```python
from build123d import *

# Parameters (mm, degrees)
F0_W     = 117.000002
F0_H     = 72.900005
F1_DEPTH = 25
F4_D     = 5.5
F5_R     = 9.5
F6_DEPTH = 40


with BuildPart() as f1:
    # F0 (on Front) → F1 (new body)
    with BuildSketch(Plane.XZ):
        with Locations((-1.050001, 2.849999)):
            Rectangle(F0_W, F0_H)
    extrude(amount=F1_DEPTH)

    # F4 (through all)
    with Locations(Plane(origin=(48.375001, 0, 48.375001), x_dir=(0.707107, 0, -0.707107), z_dir=(0.707107, 0, 0.707107))):
        with Locations((13.142212, -14.138062)):
            Hole(F4_D / 2)

    # F5 (on face) → F6 (cut)
    with BuildSketch(Plane.XZ.offset(25)):
        with Locations((-39.750002, -15.600001)):
            Circle(F5_R)
    extrude(amount=-F6_DEPTH, mode=Mode.SUBTRACT)


solid = f1.part
```
Geometry: final body of the model. Coordinates: model frame, mm. Round coordinates to 2 decimals unless told otherwise and drop trailing zeros. Loops run counter-clockwise (first coordinate to the right, second up) from the corner with the lowest first, then second, coordinate; pieces in that order, holes last.
Item 1: Mould query, pull axis Y, two halves, no side actions, for faces 1 (the flat face through (-2, 0, 3)), 2 (the cylindrical face through (17.98, -13.31, 3.1)), 3 (the cylindrical face through (-49.24, -12.68, -15.18)). Classes: released by +Y, released by -Y, zero draft, split by the parting line, or undercut.
Checked values:
face 1: released by +Y
face 2: undercut
face 3: zero draft
Item 2: Section A-A, the plane y = -12.75. Output: boundary loops of the cut face in (x, z), plus the area to 3 significant figures.
Checked values:
outline: (-59.55, -33.6) - (-18.37, -33.6) - (54.53, 39.3) - (-59.55, 39.3) - close; (-11.66, -33.6) - (57.45, -33.6) - (57.45, 35.51) - close; hole circle Ø19 at (-39.75, -15.6)
area: 7,760 mm2
Item 3: Section B-B, the plane x = -33. Output: boundary loops of the cut face in (y, z), plus the area to 3 significant figures.
Checked values:
outline: (-25, -33.6) - (0, -33.6) - (0, -22.28) - (-25, -22.28) - close; (-25, -8.92) - (0, -8.92) - (0, 39.3) - (-25, 39.3) - close
area: 1,490 mm2
Item 4: Section C-C, the plane y = -6.5. Output: boundary loops of the cut face in (x, z), plus the area to 3 significant figures.
Checked values:
outline: (-59.55, -33.6) - (57.45, -33.6) - (57.45, 39.3) - (-59.55, 39.3) - close; hole circle Ø19 at (-39.75, -15.6)
area: 8,250 mm2
Item 5: Line query: L1, parallel to X at y = -15.75, z = -12; L2, parallel to X at y = -13, z = -22; L3, parallel to X at y = -2.5, z = -22. Output: solid intervals per line, ascending.
Checked values:
L1: x = -59.55 to -48.54, -30.96 to 3.43, 9.74 to 57.45
L2: x = -59.55 to -46.77, -32.73 to -6.95, 0.13 to 57.45
L3: x = -59.55 to -46.77, -32.73 to 57.45
Item 6: Section D-D, the plane z = -22.5. State how many separate pieces and enclosed holes the cut face has, plus the area to 3 significant figures.
Checked values:
separate pieces: 2
enclosed holes: 1
area: 2,560 mm2
